from build123d import *

# Parameters (mm, degrees)
F0_R     = 12.5
F1_DEPTH = 5
F2_R     = 4
F3_DEPTH = 20
F4_SIZE2 = 4
F4_SIZE  = 1
F5_R     = 1.75
F6_DEPTH = 24


with BuildPart() as f1:
    # F0 (on Top) → F1 (new body)
    with BuildSketch(Plane.XY):
        Circle(F0_R)
    extrude(amount=F1_DEPTH)

    # F2 (on face) → F3 (join)
    with BuildSketch(Plane.XY.offset(5)):
        Circle(F2_R)
    extrude(amount=F3_DEPTH)

    # F4
    f4_edges = [f1.edges().sort_by_distance(p)[0] for p in [
        (-4, 0, 25),
    ]]
    f4_side = f1.faces().sort_by_distance((0, 0, 25))[0]
    chamfer(f4_edges, length=F4_SIZE, length2=F4_SIZE2, reference=f4_side)

    # F5 (on face) → F6 (cut)
    with BuildSketch(Plane(origin=(0, 0, 0), x_dir=(1, 0, 0), z_dir=(0, 0, -1))):
        Circle(F5_R)
    extrude(amount=-F6_DEPTH, mode=Mode.SUBTRACT)


solid = f1.part
Work out the finished part from the listing and answer in its coordinate system (mm). A direction names the side the tool comes from. Round coordinates to 2 decimals unless told otherwise and drop trailing zeros. Loops run counter-clockwise (first coordinate to the right, second up) from the corner with the lowest first, then second, coordinate; pieces in that order, holes last. Notation, with made-up numbers: (54.5, 77) - (78.5, 77) arc R27 ccw to (78.5, 105) - close; hole circle Ø4 at (48.25, -32.5). An arc over 180 degrees is marked (long way). One line per item, written item: value.
Q1. Find section A-A on x = 0. Give the vertices of the cut face in (y, z).
Check values:
outline: (-12.5, 0) - (-1.75, 0) - (-1.75, 24) - (1.75, 24) - (1.75, 0) - (12.5, 0) - (12.5, 5) - (4, 5) - (4, 21) - (3, 25) - (-3, 25) - (-4, 21) - (-4, 5) - (-12.5, 5) - close
Q2. Straight lines are drawn through the part: probe 1 along Y at (x, z) = (0, 17.5); probe 2 along Z at (x, y) = (5.25, 7.25); probe 3 along Y at (x, z) = (4.5, 3). For each, find the intervals that lie inside material, in ascending order.
Check values:
probe 1: -4 to -1.75, 1.75 to 4
probe 2: 0 to 5
probe 3: -11.66 to 11.66
Q3. Find section C-C on z = 15.25. Give the vertices of the cut face in (x, y), and give its area (3 significant figures).
Check values:
outline: circle Ø8 at (0, 0); hole circle Ø3.5 at (0, 0)
area: 40.6 mm2
Q4. Each of these flat-tipped pins is pushed along its axis until it touches: pin 1 Ø1.5 at (y, z) = (4, 20) entering from -X; pin 2 Ø3 at (x, y) = (8, 7) entering from +Z. Where does it stop, or does it pass through?
Check values:
pin 1: x = -2.33
pin 2: z = 5
Q5. Find section D-D on x = 4.5. Give the vertices of the cut face in (y, z), and give its area (3 significant figures).
Check values:
outline: (-11.66, 0) - (11.66, 0) - (11.66, 5) - (-11.66, 5) - close
area: 117 mm2
Q6. The mould has two halves that part along X. Classify faces 4 (the flat face through (0, 0, 25)), 5 (the cylindrical face through (11.923, 3.755, 2.465)), 6 (the cylindrical face through (1.617, 0.67, 11.832)): +X half, -X half, draft (parallel to the pull), parting line (faces both ways), or undercut.
Check values:
face 4: draft
face 5: parting line
face 6: undercut
Q7. For faces 1 (the flat face through (0, -3, 0)), 2 (the flat face through (0, 0, 24)), 3 (the cylindrical face through (-0.867, -3.905, 12.888)), determine the directions among +Z, -Z, +X, -X, +Y, -Y from which every point of the face is accessible in a straight line to the end or side of a thin tool.
Check values:
face 1: -Z, +X, -X, +Y, -Y
face 2: -Z
face 3: +Z
